Check sheet for the modelled part. Datum: model origin and axes. Units: mm. A direction names the side the tool comes from. Round coordinates to 2 decimals unless told otherwise and drop trailing zeros. Write each loop counter-clockwise with the first axis right and the second up, starting at its lowest first coordinate (ties: lowest second). Pieces come first, ordered by that corner, then holes. Notation, with made-up numbers: (43, 31) -> (90, 31) arc R16 ccw to (90, 42) -> close; hole circle Ø1 at (13, 58.5). An arc over 180 degrees is marked (long way). Answer as a JSON object with one key per item and string values. Group by question number.
```python
from build123d import *

# Parameters (mm, degrees)
SKETCH4_W                               = 180
SKETCH4_H                               = 180
BOSS_EXTRUDE2_DEPTH                     = 10
SKETCH5_R                               = 70
BOSS_EXTRUDE3_DEPTH                     = 80
SKETCH6_W                               = 80
SKETCH6_H                               = 40
BOSS_EXTRUDE4_DEPTH                     = 100
SKETCH7_R                               = 65
CUT_EXTRUDE1_DEPTH                      = 3
CBORE_FOR_M6_HEX_HEAD_BOLT2_D           = 6.6
CBORE_FOR_M6_HEX_HEAD_BOLT2_CBORE_D     = 14.55
CBORE_FOR_M6_HEX_HEAD_BOLT2_CBORE_DEPTH = 4.38
FILLET1_R                               = 10
FILLET2_R                               = 10
FILLET3_R                               = 2


with BuildPart() as part:
    # Sketch4 → Boss-Extrude2 (new body)
    with BuildSketch(Plane(origin=(0, 0, 0), x_dir=(1, 0, 0), z_dir=(0, 1, 0))):
        Rectangle(SKETCH4_W, SKETCH4_H)
    extrude(amount=BOSS_EXTRUDE2_DEPTH)

    # Sketch5 → Boss-Extrude3 (add)
    with BuildSketch(Plane(origin=(0, 10, 0), x_dir=(1, 0, 0), z_dir=(0, 1, 0))):
        with Locations(Location((0, 0, 0), (0, 0, 270))):
            Circle(SKETCH5_R)
    extrude(amount=BOSS_EXTRUDE3_DEPTH)

    # Sketch6 → Boss-Extrude4 (add)
    with BuildSketch(Plane.XY):
        with Locations((0, 50)):
            Rectangle(SKETCH6_W, SKETCH6_H)
    extrude(amount=BOSS_EXTRUDE4_DEPTH)

    # Sketch7 → Cut-Extrude1 (cut)
    with BuildSketch(Plane(origin=(0, 90, 0), x_dir=(1, 0, 0), z_dir=(0, 1, 0))):
        with Locations(Location((0, 0, 0), (0, 0, 270))):
            Circle(SKETCH7_R)
    extrude(amount=-CUT_EXTRUDE1_DEPTH, mode=Mode.SUBTRACT)

    # CBORE for M6 Hex Head Bolt2 (through all)
    with Locations(Plane(origin=(0, 10, 0), x_dir=(1, 0, 0), z_dir=(0, 1, 0))):
        with Locations((-75, 75), (75, 75), (75, -75), (-75, -75)):
            CounterBoreHole(CBORE_FOR_M6_HEX_HEAD_BOLT2_D / 2, CBORE_FOR_M6_HEX_HEAD_BOLT2_CBORE_D / 2, CBORE_FOR_M6_HEX_HEAD_BOLT2_CBORE_DEPTH)

    # Fillet1
    fillet1_edges = [part.edges().sort_by_distance(p)[0] for p in [
        (90, 5, 90),
        (-90, 5, 90),
        (-90, 5, -90),
        (90, 5, -90),
    ]]
    fillet(fillet1_edges, radius=FILLET1_R)

    # Fillet2
    fillet2_edges = [part.edges().sort_by_distance(p)[0] for p in [
        (-40, 70, 78.722813233),
        (40, 30, 78.722813233),
        (-40, 30, 78.722813233),
        (40, 70, 78.722813233),
    ]]
    fillet(fillet2_edges, radius=FILLET2_R)

    # Fillet3
    fillet3_edges = [part.edges().sort_by_distance(p)[0] for p in [
        (-15.375488216, 70, 68.290514437),
        (-36.872641972, 32.735924536, 59.501330019),
        (36.872641972, 32.735924536, 59.501330019),
        (-36.872641975, 67.264075467, 59.501330017),
        (36.872641972, 67.264075464, 59.501330019),
        (0, 10, -70),
        (90, 10, 0),
        (0, 10, 90),
        (0, 10, -90),
        (-90, 10, 0),
        (-87.071067812, 10, 87.071067812),
        (87.071067812, 10, -87.071067812),
        (-87.071067812, 10, -87.071067812),
        (87.071067812, 10, 87.071067812),
        (15.375488216, 30, 68.290514437),
        (0, 30, 100),
        (-40, 50, 57.445626465),
        (-40, 50, 100),
        (40, 50, 100),
        (0, 70, 100),
        (37.071067812, 67.071067812, 100),
        (-37.071067812, 67.071067812, 100),
        (37.071067812, 32.928932188, 100),
        (-37.071067812, 32.928932188, 100),
        (40, 50, 57.445626465),
    ]]
    fillet(fillet3_edges, radius=FILLET3_R)


solid = part.part
```
(1) Scan lines: line 1 along Z through (x, y) = (75, 8) (3 decimals); line 2 along Z through (x, y) = (-75, 3.3). Record each from-to range of solid material in increasing order.
(2) Access from +Z, -Z, +X, -X, +Y, -Y to the whole of each face (thin tool, end or side, straight path). Record for faces 4 (the cylindrical face through (77.43, 2.77, -77.23)), 5 (the cylindrical face through (36.99, 67.15, 78.52)), 6 (the cylindrical face through (-36.99, 32.85, 78.52)), 7 (the cylindrical face through (81.72, 7.84, -72.21)), 8 (the flat face through (-61.9, 90, 20.4)).
(3) Section check C-C on z = 75. State how many separate pieces and enclosed holes the cut face has, then the cut area to 3 significant figures.
(4) Section check A-A on z = -75. Record the cut outline in (x, y) (3 decimals).
(5) Section check B-B on x = 75. Record the cut outline in (y, z) (3 decimals).
(6) Section check D-D on y = 54. Record the cut outline in (x, z), then the cut area to 3 significant figures.
(7) Release check for a two-part mould opening along X. For faces 1 (the flat face through (-90, 4, 1)), 2 (the flat face through (-40.3, 10, -59.9)), 3 (the flat face through (78, 5.62, 77)) record: pulls with the +X half, pulls with the -X half, needs draft (parallel to the pull), parting line crosses it, or undercut.
(8) Go/stop test with flat-tipped pins: pin 1 Ø19 at (x, z) = (75, 75) entering from -Y; pin 2 Ø16.5 at (x, z) = (-75, -75) entering from +Y; pin 3 Ø1 at (y, z) = (38.5, -40.5) entering from -X; pin 4 Ø4 at (x, y) = (61.5, 41.5) entering from -Z. Record where each tip stops, or that it passes through.
Data:
{
 "1": {"line 1": "z = -90 to -82.275, -67.725 to 67.725, 82.275 to 90", "line 2": "z = -90 to -78.3, -71.7 to 71.7, 78.3 to 90"},
 "2": {"face 4": "+Y, -Y", "face 5": "+Z, +X, +Y", "face 6": "+Z, -X", "face 7": "+Y", "face 8": "+Z, -Z, +X, -X, +Y"},
 "3": {"separate pieces": "4", "enclosed holes": "0", "area": "4,710 mm²"},
 "4": {"outline": "(-90, 0) -> (-78.3, 0) -> (-78.3, 5.62) -> (-82.275, 5.62) -> (-82.275, 10) -> (-88, 10) arc R2 ccw to (-90, 8) -> close; (-71.7, 0) -> (71.7, 0) -> (71.7, 5.62) -> (67.725, 5.62) -> (67.725, 10) -> (-67.725, 10) -> (-67.725, 5.62) -> (-71.7, 5.62) -> close; (78.3, 0) -> (90, 0) -> (90, 8) arc R2 ccw to (88, 10) -> (82.275, 10) -> (82.275, 5.62) -> (78.3, 5.62) -> close"},
 "5": {"outline": "(0, -90) -> (8, -90) arc R2 ccw to (10, -88) -> (10, -82.275) -> (5.62, -82.275) -> (5.62, -78.3) -> (0, -78.3) -> close; (0, -71.7) -> (5.62, -71.7) -> (5.62, -67.725) -> (10, -67.725) -> (10, 67.725) -> (5.62, 67.725) -> (5.62, 71.7) -> (0, 71.7) -> close; (0, 78.3) -> (5.62, 78.3) -> (5.62, 82.275) -> (10, 82.275) -> (10, 88) arc R2 ccw to (8, 90) -> (0, 90) -> close"},
 "6": {"outline": "(-40.83, 56.86) arc R70 ccw (long way) to (40.83, 56.86) arc R2 cw to (40, 58.48) -> (40, 98) arc R2 ccw to (38, 100) -> (-38, 100) arc R2 ccw to (-40, 98) -> (-40, 58.48) arc R2 cw to start", "area": "18,100 mm²"},
 "7": {"face 1": "pulls with the -X half", "face 2": "needs draft", "face 3": "undercut"},
 "8": {"pin 1": "stops at y = 0", "pin 2": "stops at y = 10", "pin 3": "stops at x = -57.45", "pin 4": "stops at z = -36.87"}
}
